Geometry check sheet. Reference: the model listing, model coordinates, mm. Give positions to 0.01 mm unless a question says otherwise; leave off trailing zeros. Write each loop counter-clockwise with the first axis right and the second up, starting at its lowest first coordinate (ties: lowest second). Pieces come first, ordered by that corner, then holes. Notation, with made-up numbers: M -26,42.5 L -18,42.5 A14 cw -18,50.5 Z; hole C 17,77 d9. An arc over 180 degrees is marked long. One line per item, written item: value. Start each with the question number.
1. Gauge pin test, flat ends, axial feed: pin 1 (1.5 mm diameter, centred on y = 46.5, z = 8, fed in from +X); pin 2 (1.5 mm diameter, centred on x = -4, y = 45.5, fed in from -Z); pin 3 (1.5 mm diameter, centred on y = 46.5, z = -4, fed in from +X). Record the tip position at first contact, or that the pin passes through.
2. Cross-section at D-D on x = -1.75. Record the cut outline in (y, z).
3. Cross-section at B-B on z = 20. Record the cut outline in (x, y).
4. Scan lines: line 1 (Z direction, x = -3.5, y = 48.75); line 2 (X direction, y = 47.8, z = 21); line 3 (Y direction, x = -0.75, z = -7.5). Record each from-to range of solid material in increasing order.
5. Cross-section at A-A on z = 37. Record the cut outline in (x, y).
6. Cross-section at C-C on x = 2.5. Record the cut outline in (y, z).
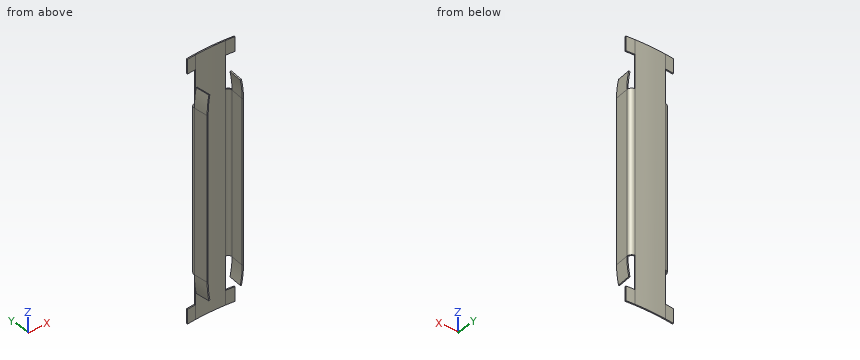
from build123d import *

# Parameters (mm, degrees)
EXTRUSION1_DEPTH = 34
EXTRUSION2_DEPTH = 3
EXTRUSION3_START = 10
EXTRUSION3_DEPTH = 10
EXTRUSION4_DEPTH = 10
EXTRUSION5_START = -3
EXTRUSION5_DEPTH = 3
EXTRUSION6_DEPTH = 3


with BuildPart() as part:
    # Esquisse1 → Extrusion1 (new body)
    with BuildSketch(Plane.XY):
        with BuildLine():
            Line((-3.933519007, 47.82875629), (-3.672032862, 44.839955984))
            Line((-3.672032862, 44.839955984), (-3.921081537, 44.818167048))
            Line((-3.921081537, 44.818167048), (-4.182567681, 47.806967354))
            ThreePointArc((-4.182567681, 47.806967354), (-3.945679792, 48.544855891), (-3.252755753, 48.891917328))
            ThreePointArc((-3.252755753, 48.891917328), (-1.627275473, 48.972971878), (0, 49))
            Line((0, 49), (0, 48.75))
            ThreePointArc((0, 48.75), (-1.618973047, 48.723109776), (-3.236160061, 48.64246877))
            ThreePointArc((-3.236160061, 48.64246877), (-3.75585309, 48.382172692), (-3.933519007, 47.82875629))
        make_face()
    extrusion1 = extrude(amount=EXTRUSION1_DEPTH)

    # Esquisse2 → Extrusion2 (add)
    with BuildSketch(Plane(origin=(-3.921081537, 44.818167048, 0), x_dir=(0.9961946980917463, 0.08715574274764933, 0), z_dir=(0.08715574274764933, -0.9961946980917464, 0))):
        with BuildLine():
            Line((0, 34), (0.25, 34))
            ThreePointArc((0.25, 34), (0.350010978, 35.985052), (0.649031032, 37.95))
            Line((0.649031032, 37.95), (0.404082058, 38))
            ThreePointArc((0.404082058, 38), (0.10127694, 36.01017924), (0, 34))
        make_face()
        with BuildLine():
            Line((0.404082058, -4), (0.649031032, -3.95))
            ThreePointArc((0.649031032, -3.95), (0.350010978, -1.985052), (0.25, 0))
            Line((0.25, 0), (0, 0))
            ThreePointArc((0, 0), (0.10127694, -2.01017924), (0.404082058, -4))
        make_face()
    extrusion2 = extrude(amount=-EXTRUSION2_DEPTH)

    # Esquisse3 → Extrusion3 (add)
    with BuildSketch(Plane(origin=(0, 0, 0), x_dir=(-1, 0, 0), z_dir=(0, 0, -1)).offset(EXTRUSION3_START)):
        with BuildLine():
            Line((3.236160061, 48.64246877), (3.252755753, 48.891917328))
            ThreePointArc((3.252755753, 48.891917328), (1.627275473, 48.972971878), (0, 49))
            Line((0, 49), (0, 48.75))
            ThreePointArc((0, 48.75), (1.618973047, 48.723109776), (3.236160061, 48.64246877))
        make_face()
    extrusion3 = extrude(amount=-EXTRUSION3_DEPTH)

    # Esquisse4 → Extrusion4 (add)
    with BuildSketch(Plane.XY.offset(34)):
        with BuildLine():
            Line((-3.236160061, 48.64246877), (-3.252755753, 48.891917328))
            ThreePointArc((-3.252755753, 48.891917328), (-1.627275473, 48.972971878), (0, 49))
            Line((0, 49), (0, 48.75))
            ThreePointArc((0, 48.75), (-1.618973047, 48.723109776), (-3.236160061, 48.64246877))
        make_face()
    extrusion4 = extrude(amount=EXTRUSION4_DEPTH)

    # Esquisse5 → Extrusion5 (add)
    with BuildSketch(Plane.XY.offset(44).offset(EXTRUSION5_START)):
        with BuildLine():
            Line((-5.1218947, 48.731572873), (-5.095762584, 48.482942399))
            ThreePointArc((-5.095762584, 48.482942399), (-2.551377867, 48.683189819), (0, 48.75))
            Line((0, 48.75), (0, 49))
            ThreePointArc((0, 49), (-2.564461856, 48.932847203), (-5.1218947, 48.731572873))
        make_face()
    extrusion5 = extrude(amount=EXTRUSION5_DEPTH)

    # Esquisse6 → Extrusion6 (add)
    with BuildSketch(Plane(origin=(0, 0, -10), x_dir=(-1, 0, 0), z_dir=(0, 0, -1))):
        with BuildLine():
            Line((0, 49), (0, 48.75))
            ThreePointArc((0, 48.75), (2.551377867, 48.683189819), (5.095762584, 48.482942399))
            Line((5.095762584, 48.482942399), (5.1218947, 48.731572873))
            ThreePointArc((5.1218947, 48.731572873), (2.564461856, 48.932847203), (0, 49))
        make_face()
    extrusion6 = extrude(amount=-EXTRUSION6_DEPTH)

    # Symétrie1: Extrusion1, Extrusion2, Extrusion3, Extrusion4, Extrusion5, Extrusion6 across plane
    add(extrusion1.mirror(Plane(origin=(0, 48.75, 34), x_dir=(0, 0, 1), z_dir=(-1, 0, 0))))
    add(extrusion2.mirror(Plane(origin=(0, 48.75, 34), x_dir=(0, 0, 1), z_dir=(-1, 0, 0))))
    add(extrusion3.mirror(Plane(origin=(0, 48.75, 34), x_dir=(0, 0, 1), z_dir=(-1, 0, 0))))
    add(extrusion4.mirror(Plane(origin=(0, 48.75, 34), x_dir=(0, 0, 1), z_dir=(-1, 0, 0))))
    add(extrusion5.mirror(Plane(origin=(0, 48.75, 34), x_dir=(0, 0, 1), z_dir=(-1, 0, 0))))
    add(extrusion6.mirror(Plane(origin=(0, 48.75, 34), x_dir=(0, 0, 1), z_dir=(-1, 0, 0))))


solid = part.part
Report:
1. pin 1: stops at x = 4.13
1. pin 2: stops at z = -4
1. pin 3: stops at x = 3.82
2. outline: M 48.72,-10 L 48.97,-10 L 48.97,44 L 48.72,44 Z
3. outline: M -4.18,47.81 L -3.92,44.82 L -3.67,44.84 L -3.93,47.83 A0.75 cw -3.24,48.64 A48.75 cw 3.24,48.64 A0.75 cw 3.93,47.83 L 3.67,44.84 L 3.92,44.82 L 4.18,47.81 A1 ccw 3.25,48.89 A49 ccw -3.25,48.89 A1 ccw Z
4. line 1: z = -10 to -7, 0 to 34, 41 to 44
4. line 2: x = -4.18 to -3.93, 3.93 to 4.18
4. line 3: y = 48.74 to 48.99
5. outline: M -3.96,47.83 L -3.7,44.84 L -3.44,44.86 L -3.71,47.85 Z; M -3.25,48.89 L -3.24,48.64 A48.75 cw 3.24,48.64 L 3.25,48.89 A49 ccw Z; M 3.44,44.86 L 3.7,44.84 L 3.96,47.83 L 3.71,47.85 Z
6. outline: M 48.69,-10 L 48.94,-10 L 48.94,44 L 48.69,44 Z
